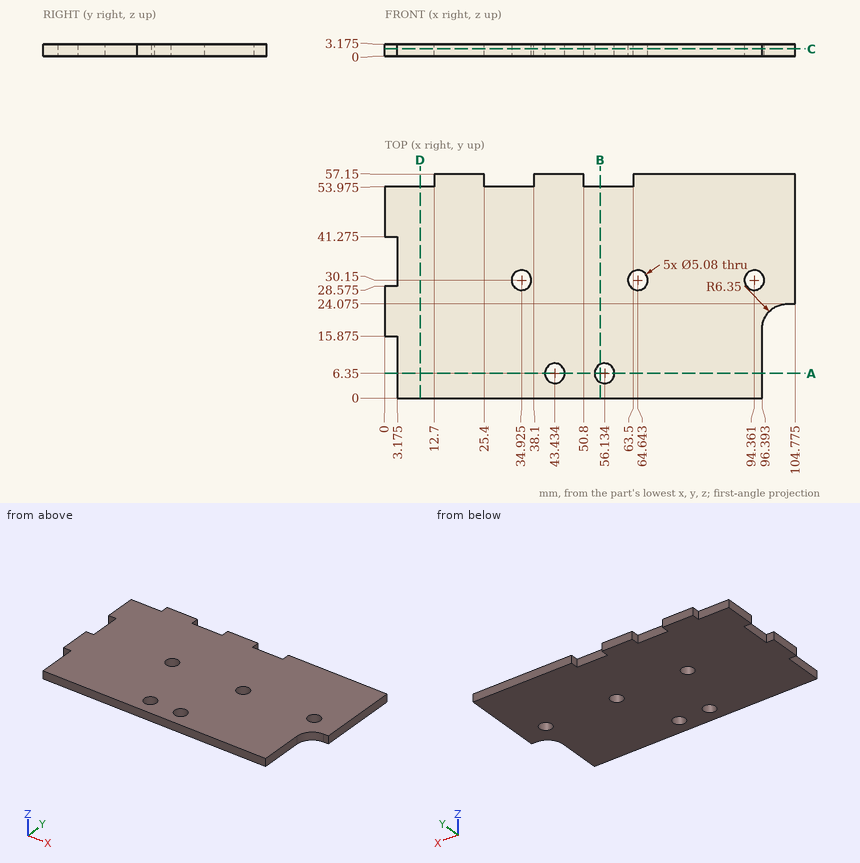
Drawing for the job (mm, zero at the part's lowest x, y, z). Round coordinates to 2 decimals unless told otherwise and drop trailing zeros. Loops run counter-clockwise (first coordinate to the right, second up) from the corner with the lowest first, then second, coordinate; pieces in that order, holes last.
1. Band-saw the part on B-B, the plane x = 55. List the corners of the cut face in (y, z) (1 decimal), and give its area (3 significant figures).
Check values:
outline: (0, 0) - (4.1, 0) - (4.1, 3.2) - (0, 3.2) - close; (8.6, 0) - (54, 0) - (54, 3.2) - (8.6, 3.2) - close
area: 157 mm2
2. Band-saw the part on A-A, the plane y = 6.35. List the corners of the cut face in (x, z) (3 decimals).
Check values:
outline: (3.175, 0) - (40.894, 0) - (40.894, 3.175) - (3.175, 3.175) - close; (45.974, 0) - (53.594, 0) - (53.594, 3.175) - (45.974, 3.175) - close; (58.674, 0) - (96.393, 0) - (96.393, 3.175) - (58.674, 3.175) - close
3. Drop flat-ended pins along their axis: P1, Ø1, axis at y = 35, z = 1.5, coming from the -X side (3 decimals); P2, Ø3, axis at x = 43.434, y = 6.35, coming from the +Z side; P3, Ø1, axis at x = 1, z = 2.5, coming from the -Y side (3 decimals); P4, Ø1, axis at x = 104, z = 2.5, coming from the -Y side (3 decimals). Give the stop position or say it passes through.
Check values:
P1: stops at x = 3.175
P2: passes through
P3: stops at y = 15.875
P4: stops at y = 24.075
4. Band-saw the part on C-C, the plane z = 1.9. Count the separate pieces of the cut face and the enclosed holes in it, and give its area (3 significant figures).
Check values:
separate pieces: 1
enclosed holes: 5
area: 5,480 mm2
5. Band-saw the part on D-D, the plane x = 9. List the corners of the cut face in (y, z) (3 decimals).
Check values:
outline: (0, 0) - (53.975, 0) - (53.975, 3.175) - (0, 3.175) - close
6. Wall check: probe 1 along X at (y, z) = (54.5, 2.05) (3 decimals); probe 2 along X at (y, z) = (7, 0.2) (1 decimal); probe 3 along X at (y, z) = (16.5, 1.3). Give the ranges that are in metal, low to high.
Check values:
probe 1: x = 12.7 to 25.4, 38.1 to 50.8, 63.5 to 104.775
probe 2: x = 3.2 to 41, 45.9 to 53.7, 58.6 to 96.4
probe 3: x = 0 to 96.39
